```python
from build123d import *

# Parameters (mm, degrees)
ESQUISSE1_W             = 100
ESQUISSE1_H             = 55
BOSS_EXTRU_1_DEPTH      = 35
ESQUISSE2_W             = 29.5
ESQUISSE2_H             = 2.5
ENL_V_MAT_EXTRU_1_DEPTH = 20


with BuildPart() as part:
    # Esquisse1 → Boss.-Extru.1 (new body)
    with BuildSketch(Plane.XY):
        Rectangle(ESQUISSE1_W, ESQUISSE1_H)
    extrude(amount=BOSS_EXTRU_1_DEPTH)

    # Esquisse2 → Enlèv. mat.-Extru.1 (cut)
    with BuildSketch(Plane.XY.offset(35)):
        with BuildLine():
            Line((-9.5, 4.5), (-9.5, -4.5))
            ThreePointArc((-9.5, -4.5), (0, -5.06418194), (9.5, -4.5))
            Line((9.5, -4.5), (9.5, 4.5))
            ThreePointArc((9.5, 4.5), (0, 5.06418194), (-9.5, 4.5))
        make_face()
        with Locations((0, 13.607565721)):
            Rectangle(ESQUISSE2_W, ESQUISSE2_H)
    extrude(amount=-ENL_V_MAT_EXTRU_1_DEPTH, mode=Mode.SUBTRACT)


solid = part.part
```
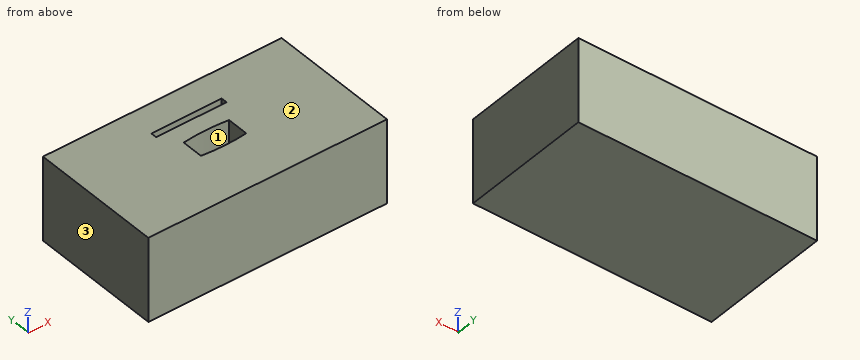
Part model, mm, in its own coordinate system. Face numbers are marked on the shaded views. Round coordinates to 2 decimals unless told otherwise and drop trailing zeros. Write each loop counter-clockwise with the first axis right and the second up, starting at its lowest first coordinate (ties: lowest second). Pieces come first, ordered by that corner, then holes.
Item 1: Cut at C-C, the plane x = 1. Give the cut face in (y, z).
Results:
outline: (-27.5, 0) - (27.5, 0) - (27.5, 35) - (14.86, 35) - (14.86, 15) - (12.36, 15) - (12.36, 35) - (5.06, 35) - (5.06, 15) - (-5.06, 15) - (-5.06, 35) - (-27.5, 35) - close
Item 2: Cut at B-B, the plane y = 13.5. Give the cut face in (x, z).
Results:
outline: (-50, 0) - (50, 0) - (50, 35) - (14.75, 35) - (14.75, 15) - (-14.75, 15) - (-14.75, 35) - (-50, 35) - close
Item 3: Probe L1, parallel to Y at x = -9, z = 30; L2, parallel to X at y = 4, z = 27. List the from-to ranges inside material, lowest first.
Results:
L1: y = -27.5 to -4.56, 4.56 to 12.36, 14.86 to 27.5
L2: x = -50 to -9.5, 9.5 to 50
Item 4: Two-plate mould, pull along X, no slides. Class the marked faces 1, 2 and 3: +X half, -X half, draft (parallel to the pull), parting line (faces both ways), or undercut.
Results:
face 1: undercut
face 2: draft
face 3: -X half
Item 5: Cut at A-A, the plane z = 21. Give the cut face in (x, y), plus the area to 3 significant figures.
Results:
outline: (-50, -27.5) - (50, -27.5) - (50, 27.5) - (-50, 27.5) - close; hole (-14.75, 12.36) - (14.75, 12.36) - (14.75, 14.86) - (-14.75, 14.86) - close; hole (-9.5, -4.5) arc R80.27 ccw to (9.5, -4.5) - (9.5, 4.5) arc R80.27 ccw to (-9.5, 4.5) - close
area: 5,240 mm2
Item 6: Drop flat-ended pins along their axis: pin 1 Ø5 at (x, y) = (4.5, 1.5) entering from +Z; pin 2 Ø2 at (x, y) = (18.5, 16.5) entering from -Z. Give the stop position or say it passes through.
Results:
pin 1: stops at z = 15
pin 2: stops at z = 0
